```python
from build123d import *

# Parameters (mm, degrees)
BOSS_EXTRUDE1_DEPTH = 3
SKETCH2_R           = 1.5
CUT_EXTRUDE1_DEPTH  = 3
SKETCH6_R           = 1.5
CUT_EXTRUDE2_DEPTH  = 3
SKETCH8_W           = 60
SKETCH8_H           = 90
CUT_EXTRUDE4_DEPTH  = 3
SKETCH3_R           = 1.5
CUT_EXTRUDE5_DEPTH  = 3


with BuildPart() as part:
    # Sketch1 → Boss-Extrude1 (new body)
    with BuildSketch(Plane(origin=(0, 0, 0), x_dir=(1, 0, 0), z_dir=(0, 1, 0))):
        Polygon((-20, -130), (0, -130), (0, -105), (70, -105), (70, -130), (180, -130), (180, 70), (70, 70), (70, 45), (0, 45), (0, 70), (-20, 70), align=None)
    extrude(amount=BOSS_EXTRUDE1_DEPTH)

    # Sketch2 → Cut-Extrude1 (cut)
    with BuildSketch(Plane(origin=(0, 3, 0), x_dir=(1, 0, 0), z_dir=(0, 1, 0))):
        with Locations(Location((29.5, -96, 0), (0, 0, 270))):
            Circle(SKETCH2_R)
        with Locations(Location((29.5, -76, 0), (0, 0, 270))):
            Circle(SKETCH2_R)
        with Locations(Location((40.5, -96, 0), (0, 0, 90))):
            Circle(SKETCH2_R)
        with Locations(Location((40.5, -76, 0), (0, 0, 90))):
            Circle(SKETCH2_R)
        with Locations(Location((29.5, 36, 0), (0, 0, 90))):
            Circle(SKETCH2_R)
        with Locations(Location((40.5, 36, 0), (0, 0, 270))):
            Circle(SKETCH2_R)
        with Locations(Location((40.5, 16, 0), (0, 0, 270))):
            Circle(SKETCH2_R)
        with Locations(Location((29.5, 16, 0), (0, 0, 90))):
            Circle(SKETCH2_R)
    extrude(amount=-CUT_EXTRUDE1_DEPTH, mode=Mode.SUBTRACT)

    # Sketch6 → Cut-Extrude2 (cut)
    with BuildSketch(Plane(origin=(0, 3, 0), x_dir=(1, 0, 0), z_dir=(0, 1, 0))):
        with Locations(Location((170, -120, 0), (0, 0, 270))):
            Circle(SKETCH6_R)
        with Locations(Location((170, 60, 0), (0, 0, 90))):
            Circle(SKETCH6_R)
        with Locations(Location((90, -120, 0), (0, 0, 90))):
            Circle(SKETCH6_R)
        with Locations(Location((90, 60, 0), (0, 0, 270))):
            Circle(SKETCH6_R)
    extrude(amount=-CUT_EXTRUDE2_DEPTH, mode=Mode.SUBTRACT)

    # Sketch8 → Cut-Extrude4 (cut)
    with BuildSketch(Plane(origin=(0, 3, 0), x_dir=(1, 0, 0), z_dir=(0, 1, 0))):
        with Locations((150, -30)):
            Rectangle(SKETCH8_W, SKETCH8_H)
    extrude(amount=-CUT_EXTRUDE4_DEPTH, mode=Mode.SUBTRACT)

    # Sketch3 → Cut-Extrude5 (cut)
    with BuildSketch(Plane(origin=(0, 3, 0), x_dir=(1, 0, 0), z_dir=(0, 1, 0))):
        with Locations(Location((-10, -120, 0), (0, 0, 270))):
            Circle(SKETCH3_R)
        with Locations(Location((160, -120, 0), (0, 0, 270))):
            Circle(SKETCH3_R)
        with Locations(Location((160, 60, 0), (0, 0, 90))):
            Circle(SKETCH3_R)
        with Locations(Location((-10, 60, 0), (0, 0, 90))):
            Circle(SKETCH3_R)
    extrude(amount=-CUT_EXTRUDE5_DEPTH, mode=Mode.SUBTRACT)


solid = part.part
```
Verification items for the finished model (mm, model axes). Give positions to 0.01 mm unless a question says otherwise; leave off trailing zeros. Loops run counter-clockwise (first coordinate to the right, second up) from the corner with the lowest first, then second, coordinate; pieces in that order, holes last.
1. Go/stop test with flat-tipped pins: pin 1 Ø4 at (x, z) = (-10, -60) entering from -Y; pin 2 Ø0.9 at (x, y) = (51.5, 2) entering from +Z. Record where each tip stops, or that it passes through.
2. Section check C-C, the plane x = 53.5. Enter the section's corners in (y, z).
3. Section check B-B, the plane y = 0.6. Count the separate pieces of the cut face and the enclosed holes in it, then the cut area to 3 significant figures.
4. Thickness scan on line 1 (X direction, y = 1, z = -60); line 2 (Z direction, x = 170, y = 1.3); line 3 (Z direction, x = 162, y = 1). Record the ranges inside material, lowest first.
5. Section check A-A, the plane x = 152.5. Enter the section's corners in (y, z).
Geometry says:
1. pin 1: stops at y = 0
1. pin 2: stops at z = 105
2. outline: (0, -45) - (3, -45) - (3, 105) - (0, 105) - close
3. separate pieces: 1
3. enclosed holes: 16
3. area: 31,000 mm2
4. line 1: x = -20 to -11.5, -8.5 to 0, 70 to 88.5, 91.5 to 158.5, 161.5 to 168.5, 171.5 to 180
4. line 2: z = -70 to -61.5, -58.5 to -15, 75 to 118.5, 121.5 to 130
4. line 3: z = -70 to -15, 75 to 130
5. outline: (0, -70) - (3, -70) - (3, -15) - (0, -15) - close; (0, 75) - (3, 75) - (3, 130) - (0, 130) - close
